from build123d import *

# Parameters (mm, degrees)
F0_W     = 58.42
F0_H     = 96.52
F1_DEPTH = 2.54
F0_W_2   = 2.54
F0_H_2   = 2.54
F2_DEPTH = 31.75
F3_W     = 2.54
F3_H     = 5.08
F3_H_2   = 2.54
F3_W_2   = 10.16
F3_W_3   = 10.7568990868
F3_H_3   = 83.82
F4_DEPTH = 25.4
F5_R     = 3.96875
F5_W     = 12.7
F5_H     = 6.35
F6_DEPTH = 25.4


with BuildPart() as f1:
    # F0 (on Top) → F1 (new body)
    with BuildSketch(Plane.XY):
        Rectangle(F0_W, F0_H)
    extrude(amount=F1_DEPTH)

    # F0 (on Top) → F2 (join)
    with BuildSketch(Plane.XY):
        with Locations((-30.48, 49.53)):
            Rectangle(F0_W_2, F0_H_2)
        with Locations((0, 49.53)):
            Rectangle(F0_W, F0_H_2)
        with Locations((-30.48, 0)):
            Rectangle(F0_W_2, F0_H)
        with Locations((30.48, 49.53)):
            Rectangle(F0_W_2, F0_H_2)
        with Locations((-30.48, -49.53)):
            Rectangle(F0_W_2, F0_H_2)
        with Locations((30.48, 0)):
            Rectangle(F0_W_2, F0_H)
        with Locations((0, -49.53)):
            Rectangle(F0_W, F0_H_2)
        with Locations((30.48, -49.53)):
            Rectangle(F0_W_2, F0_H_2)
    extrude(amount=F2_DEPTH)

    # F3 (on face) → F4 (join)
    with BuildSketch(Plane.XY.offset(2.54)):
        with Locations((-27.94, 38.1)):
            Rectangle(F3_W, F3_H)
        with Locations((-27.94, 46.99)):
            Rectangle(F3_W, F3_H_2)
        with Locations((-21.59, 46.99)):
            Rectangle(F3_W_2, F3_H_2)
        with Locations((21.2915504566, 46.99)):
            Rectangle(F3_W_3, F3_H_2)
        with Locations((27.94, 46.99)):
            Rectangle(F3_W, F3_H_2)
        with Locations((27.94, 38.1)):
            Rectangle(F3_W, F3_H)
        with Locations((27.94, -6.35)):
            Rectangle(F3_W, F3_H_3)
        with Locations((-27.94, -6.35)):
            Rectangle(F3_W, F3_H_3)
    extrude(amount=F4_DEPTH)

    # F5 (on face) → F6 (cut)
    with BuildSketch(Plane.XZ.offset(50.8)):
        with Locations((-12.8904990852, 9.5123006031)):
            Circle(F5_R)
        with Locations((9.1495838234, 8.3475278727)):
            Rectangle(F5_W, F5_H)
    extrude(amount=-F6_DEPTH, mode=Mode.SUBTRACT)


solid = f1.part
Build history of the part. All positions in model axes, mm. A direction names the side the tool comes from. Round coordinates to 2 decimals unless told otherwise and drop trailing zeros. Write each loop counter-clockwise with the first axis right and the second up, starting at its lowest first coordinate (ties: lowest second). Pieces come first, ordered by that corner, then holes. Notation, with made-up numbers: (-8.5, 3) - (10.5, 3) arc R14 cw to (10.5, 23) - close; hole circle Ø9 at (2, 74.5). An arc over 180 degrees is marked (long way). Use CSV: the item, a comma, the result in double quotes.
(1) Wall check: line 1 (Y direction, x = -20, z = 7); line 2 (X direction, y = -10, z = 12); line 3 (Y direction, x = -0.5, z = 21). Give the ranges that are in metal, low to high.
Response:
line 1,"-50.8 to -48.26, 45.72 to 50.8"
line 2,"-31.75 to -26.67, 26.67 to 31.75"
line 3,"-50.8 to -48.26, 48.26 to 50.8"
(2) Mould opens along Y. For faces 1 (the flat face through (29.21, 10, 29)), 2 (the flat face through (-23, 45.72, 15)), 3 (the flat face through (2.8, -50, 8)) say: pulls with the +Y half, pulls with the -Y half, needs draft (parallel to the pull), parting line crosses it, or undercut.
Response:
face 1,"undercut"
face 2,"undercut"
face 3,"needs draft"
(3) Band-saw the part on B-B (z = 16.5). Write the cut outline in (x, y).
Response:
outline,"(-31.75, -50.8) - (31.75, -50.8) - (31.75, 50.8) - (-31.75, 50.8) - close; hole (-29.21, 40.64) - (-26.67, 40.64) - (-26.67, -48.26) - (26.67, -48.26) - (26.67, 40.64) - (29.21, 40.64) - (29.21, 45.72) - (15.91, 45.72) - (15.91, 48.26) - (-16.51, 48.26) - (-16.51, 45.72) - (-29.21, 45.72) - close"
(4) Band-saw the part on A-A (x = 6). Write the cut outline in (y, z).
Response:
outline,"(-50.8, 0) - (50.8, 0) - (50.8, 31.75) - (48.26, 31.75) - (48.26, 2.54) - (-48.26, 2.54) - (-48.26, 5.17) - (-50.8, 5.17) - close; (-50.8, 11.52) - (-48.26, 11.52) - (-48.26, 31.75) - (-50.8, 31.75) - close"
(5) Pin check, flat tips, straight feed: P1, Ø6.5, axis at x = -12.89, z = 9.51, coming from the -Y side; P2, Ø3, axis at x = 27.5, y = 14.5, coming from the +Z side; P3, Ø12, axis at x = -15.5, y = -0.5, coming from the +Z side. Stop position of each tip, or through.
Response:
P1,"y = 48.26"
P2,"z = 27.94"
P3,"z = 2.54"
(6) Band-saw the part on D-D (z = 8.5). Write the cut outline in (x, y).
Response:
outline,"(-31.75, -50.8) - (-16.73, -50.8) - (-16.73, -48.26) - (-26.67, -48.26) - (-26.67, 40.64) - (-29.21, 40.64) - (-29.21, 45.72) - (-16.51, 45.72) - (-16.51, 48.26) - (15.91, 48.26) - (15.91, 45.72) - (29.21, 45.72) - (29.21, 40.64) - (26.67, 40.64) - (26.67, -48.26) - (15.5, -48.26) - (15.5, -50.8) - (31.75, -50.8) - (31.75, 50.8) - (-31.75, 50.8) - close; (-9.05, -50.8) - (2.8, -50.8) - (2.8, -48.26) - (-9.05, -48.26) - close"
(7) 3-axis set-ups, long thin cutter, end or side, ignore diameter. For faces 4 (the flat face through (28, -3, 27.94)), 5 (the flat face through (-31, 0, 31.75)), 6 (the flat face through (9, -50, 11.523)): which of +Z, -Z, +X, -X, +Y, -Y reach the whole face in a straight line?
Response:
face 4,"+Z"
face 5,"+Z, +X, -X, +Y, -Y"
face 6,"-Y"
(8) Band-saw the part on C-C (y = -21). Write the cut outline in (x, z), plus the area to 3 significant figures.
Response:
outline,"(-31.75, 0) - (31.75, 0) - (31.75, 31.75) - (29.21, 31.75) - (29.21, 27.94) - (26.67, 27.94) - (26.67, 2.54) - (-26.67, 2.54) - (-26.67, 27.94) - (-29.21, 27.94) - (-29.21, 31.75) - (-31.75, 31.75) - close"
area,"439 mm²"
